For this review, take the finished solid that the model builds, in its own axes (mm). A direction names the side the tool comes from. Round coordinates to 2 decimals unless told otherwise and drop trailing zeros. Order: outer loops, then holes, each group sorted by start corner. A loop starts at its lowest first (then second) coordinate and runs counter-clockwise, first axis right, second up. Notation, with made-up numbers: M 77.5,-23.5 L 127.5,-23.5 A24 cw 127.5,1.5 Z; hole C 10,-9.75 d4. An arc over 180 degrees is marked long. Put each result on its own line as item: value.
from build123d import *

# Parameters (mm, degrees)
BOSS_EXTRUDE1_DEPTH     = 8
CUT_EXTRUDE6_DEPTH      = 169.285043392
CUT_EXTRUDE6_DEPTH_BACK = 8
SKETCH6_R               = 4.004848267
SKETCH6_R_2             = 1.500740619
SKETCH6_R_3             = 1.502884449
SKETCH6_R_4             = 1.495453733
SKETCH6_R_5             = 1.501499852
SKETCH6_R_6             = 1.504449493
SKETCH6_R_7             = 1.503694776
SKETCH6_R_8             = 1.495371025
SKETCH6_R_9             = 1.497490914


with BuildPart() as part:
    # Sketch5 → Boss-Extrude1 (new body)
    with BuildSketch(Plane.XY):
        with BuildLine():
            Line((0, -42.218893529), (150.106998899, -42.218893529))
            Line((150.106998899, -42.218893529), (150.106998899, -51.223119472))
            Line((150.106998899, -51.223119472), (155.102889251, -51.223119472))
            Line((155.102889251, -51.223119472), (160.100118241, -51.223119472))
            Line((160.100118241, -51.223119472), (160.100118241, -3.214680099))
            Line((160.100118241, -3.214680099), (155.102889251, -3.214680099))
            Line((155.102889251, -3.214680099), (150.106998899, -3.214680099))
            Line((150.106998899, -3.214680099), (150.106998899, -12.215396897))
            Line((150.106998899, -12.215396897), (0, -12.215396897))
            ThreePointArc((0, -12.215396897), (-15.001748316, -27.217145213), (0, -42.218893529))
        make_face()
    extrude(amount=BOSS_EXTRUDE1_DEPTH)

    # Sketch6 → Cut-Extrude6 (cut, two sides: drawn at the far end of the back side and taken through both)
    with BuildSketch(Plane.XY.offset(-CUT_EXTRUDE6_DEPTH_BACK)):
        with Locations((0, -27.217145213)):
            Circle(SKETCH6_R)
        with Locations((0, -37.213991998)):
            Circle(SKETCH6_R_2)
        with Locations((0, -17.219491861)):
            Circle(SKETCH6_R_3)
        with Locations((9.996605481, -27.217145213)):
            Circle(SKETCH6_R_4)
        with Locations((-9.995878708, -27.217145213)):
            Circle(SKETCH6_R_5)
        with Locations((155.102889251, -46.721006501)):
            Circle(SKETCH6_R_6)
        with Locations((155.102889251, -7.715038498)):
            Circle(SKETCH6_R_7)
        with Locations((152.604944075, -27.217145213)):
            Circle(SKETCH6_R_8)
        with Locations((157.601503746, -27.217145213)):
            Circle(SKETCH6_R_9)
    extrude(amount=CUT_EXTRUDE6_DEPTH + CUT_EXTRUDE6_DEPTH_BACK, mode=Mode.SUBTRACT)


solid = part.part
(1) Add section A-A on x = 44.5. Give the boundary of the cut face in (y, z).
A:
outline: M -42.22,0 L -12.22,0 L -12.22,8 L -42.22,8 Z
(2) To check wall thickness, follow L1, parallel to Y at x = 124, z = 6; L2, parallel to X at y = -9, z = 2.5; L3, parallel to X at y = -44, z = 1.25. State the ranges of each line that lie inside material, in increasing order.
A:
L1: y = -42.22 to -12.22
L2: x = 150.11 to 154.32, 155.88 to 160.1
L3: x = 150.11 to 160.1
(3) For faces 4 (the face through (150.107, -47, 4)), 5 (the face through (76, -12.215, 4)), 6 (the face through (-0.2, -15.73, 3.94)), list the 3-axis set-ups (+Z, -Z, +X, -X, +Y, -Y) from which the entire face can be reached by the end or side of a thin tool; tool diameter is ignored.
A:
face 4: +Z, -Z, -X, -Y
face 5: +Z, -Z, -X, +Y
face 6: +Z, -Z
(4) Add section C-C on y = -40.5. Give the boundary of the cut face in (x, z).
A:
outline: M -6.97,0 L 160.1,0 L 160.1,8 L -6.97,8 Z
(5) Insertion check: pin 1 Ø4 at (y, z) = (-8, 5) entering from -X; pin 2 Ø1.5 at (x, z) = (16.5, 6.5) entering from +Y; pin 3 Ø2.5 at (x, z) = (38, 2) entering from -Y. Each pin has a flat end and moves straight along its axis. Give the tip position at first contact, or say it passes through.
A:
pin 1: stops at x = 150.11
pin 2: stops at y = -12.22
pin 3: stops at y = -42.22
(6) Add section B-B on z = 3.25. State how many separate pieces and enclosed holes the cut face has, then the cut area to 3 significant figures.
A:
separate pieces: 1
enclosed holes: 9
area: 5,230 mm2
(7) Draft analysis for pull direction Y (two halves, no side actions). For faces 1 (the face through (-0.521, -23.246, 3.944)), 2 (the face through (71, -27, 8)), 3 (the face through (74, -42.219, 4)), state which applies: released by +Y, released by -Y, zero draft, split by the parting line, or undercut.
A:
face 1: undercut
face 2: zero draft
face 3: released by -Y
